Here's how the part is built. I have some questions about the finished solid (model axes, mm). Round coordinates to 2 decimals unless told otherwise and drop trailing zeros. Order: outer loops, then holes, each group sorted by start corner. A loop starts at its lowest first (then second) coordinate and runs counter-clockwise, first axis right, second up.
```python
from build123d import *

# Parameters (mm, degrees)
F0_R     = 1
F1_DEPTH = 5
F3_DEPTH = 10.001
F4_R     = 0.3


with BuildPart() as f1:
    # F0 (on Front) → F1 (new body, symmetric)
    with BuildSketch(Plane.XZ):
        with BuildLine():
            Line((-2, 2), (-2, 0))
            ThreePointArc((-2, 0), (0, -2), (2, 0))
            Line((2, 0), (2, 2))
            Line((2, 2), (0, 2))
            Line((0, 2), (-2, 2))
        make_face()
        Circle(F0_R, mode=Mode.SUBTRACT)
    extrude(amount=F1_DEPTH, both=True)

    # F2 (on face) → F3 (cut, through all)
    with BuildSketch(Plane.XZ.offset(5)):
        with BuildLine():
            Line((0.875, -1.7984368212), (0, 0))
            Line((0, 0), (-0.875, -1.7984368212))
            ThreePointArc((-0.875, -1.7984368212), (0, -2), (0.875, -1.7984368212))
        make_face()
    extrude(amount=-F3_DEPTH, mode=Mode.SUBTRACT)

    # F4
    f4_edges = [f1.edges().sort_by_distance(p)[0] for p in [
        (-0.875, 0, -1.798437),
        (0.875, 0, -1.798437),
        (-1.695582, -5, -1.06066),
        (-2, -5, 1),
        (1.695582, -5, -1.06066),
        (1.695582, 5, -1.06066),
        (2, 5, 1),
        (-1.695582, 5, -1.06066),
        (-2, 5, 1),
    ]]
    fillet(f4_edges, radius=F4_R)


solid = f1.part
```
1. If we section it at D-D, the plane x = 0: Write out the boundary of the cut face in (y, z), and give its area (3 significant figures).
Evaluation:
outline: (-5, 1) - (5, 1) - (5, 2) - (-5, 2) - close
area: 10.0 mm2
2. If we section it at B-B, the plane x = 0.6: Write out the boundary of the cut face in (y, z).
Evaluation:
outline: (-5, -1.23) - (5, -1.23) - (5, -0.8) - (-5, -0.8) - close; (-5, 0.8) - (5, 0.8) - (5, 2) - (-5, 2) - close
3. If we section it at C-C, the plane z = 0.45: Write out the boundary of the cut face in (x, y).
Evaluation:
outline: (-2, -4.7) arc R0.3 ccw to (-1.7, -5) - (-0.89, -5) - (-0.89, 5) - (-1.7, 5) arc R0.3 ccw to (-2, 4.7) - close; (0.89, -5) - (1.7, -5) arc R0.3 ccw to (2, -4.7) - (2, 4.7) arc R0.3 ccw to (1.7, 5) - (0.89, 5) - close
4. I need wall thicknesses on probe 1 along X at (y, z) = (1.5, 0); probe 2 along X at (y, z) = (-4.5, 0.45); probe 3 along Z at (x, y) = (-0.1, 2.75). Which ranges of each line are inside material? Lowest first, please.
Evaluation:
probe 1: x = -2 to -1, 1 to 2
probe 2: x = -2 to -0.89, 0.89 to 2
probe 3: z = 0.99 to 2
5. If we section it at A-A, the plane y = 2: Write out the boundary of the cut face in (x, z), and give its area (3 significant figures).
Evaluation:
outline: (-2, 0) arc R2 ccw to (-1.18, -1.62) arc R0.3 ccw to (-0.73, -1.5) - (-0.44, -0.9) arc R1 cw (long way) to (0.44, -0.9) - (0.73, -1.5) arc R0.3 ccw to (1.18, -1.62) arc R2 ccw to (2, 0) - (2, 2) - (-2, 2) - close
area: 9.73 mm2
6. I'm going to push a flat-ended pin straight in: P1, Ø2, axis at y = -1.5, z = -0.5, coming from the +X side. Where does the tip first touch, or does it pass through?
Evaluation:
P1: stops at x = 2
7. If we mould it in two halves opening along X, with no side actions, what happens to faces 1 (the flat face through (-1, 5, 1)), 2 (the flat face through (2, 0, 1)), 3 (the flat face through (-2, 0, 1)), 4 (the cylindrical face through (0, 0, 1))? For each: released by +X, released by -X, zero draft, split by the parting line, or undercut.
Evaluation:
face 1: zero draft
face 2: released by +X
face 3: released by -X
face 4: undercut
